```python
from build123d import *

# Parameters (mm, degrees)
SKETCH2_W         = 19.3548
SKETCH2_H         = 2.3876
SLOT_DEPTH        = 2.2352
SKETCH3_W         = 2.1844
SKETCH3_H         = 13.2842
SKETCH4_W         = 1.0922
SKETCH4_H         = 1.0922
CIRPATTERN1_COUNT = 2
CIRPATTERN1_ANGLE = 90


with BuildPart() as part:
    # BodySke → Base-Revolve (revolve)
    with BuildSketch(Plane.XY, mode=Mode.PRIVATE) as base_revolve_sk:
        Polygon((0, 0), (0, 9.6774), (0.066909223, 9.6774), (4.191, 4.7625), (38.1, 4.7625), (38.1, 0), align=None)
    revolve(base_revolve_sk.sketch.rotate(Axis((-6.35, 0, 0), (1, 0, 0)), 90), axis=Axis((-6.35, 0, 0), (1, 0, 0)))  # turned: the seam where the file's is

    # Sketch2 → Slot (cut)
    with BuildSketch(Plane.ZY):
        Rectangle(SKETCH2_W, SKETCH2_H)
    extrude(amount=-SLOT_DEPTH, mode=Mode.SUBTRACT)

    # Sketch3 → Cross section 0
    with BuildSketch(Plane.ZY):
        Rectangle(SKETCH3_W, SKETCH3_H)
    # Sketch4 → Cross section 1
    with BuildSketch(Plane.ZY.offset(-7.9756)):
        Rectangle(SKETCH4_W, SKETCH4_H)
    cross = loft(mode=Mode.SUBTRACT)

    # CirPattern1: Cross ×2 about axis
    cirpattern1_axis = Axis((0, 0, 0), (1, 0, 0))
    for i in range(1, CIRPATTERN1_COUNT):
        add(cross.rotate(cirpattern1_axis, i * CIRPATTERN1_ANGLE / (CIRPATTERN1_COUNT - 1)), mode=Mode.SUBTRACT)


solid = part.part
```
CAD build for the part. Positions are in the model's coordinates, mm. A direction names the side the tool comes from. Coordinates: 2 decimals unless noted, no trailing zeros. Order: outer loops, then holes, each group sorted by start corner. A loop starts at its lowest first (then second) coordinate and runs counter-clockwise, first axis right, second up. Notation, with made-up numbers: M 44.25,-32 L 92.25,-32 A27 ccw 92.25,6 Z; hole C 69.25,-4 d11. An arc over 180 degrees is marked long. Answer as CSV lines item,"result".
1) Mould opens along Y. For faces 3 (the flat face through (7.976, 0, 0)), 4 (the flat face through (1, -1.194, 4)), 5 (the cylindrical face through (21.38, 4.65, -1.03)), 6 (the flat face through (38.1, 0, 0)) say: released by +Y, released by -Y, zero draft, split by the parting line, or undercut.
Verdict:
face 3,"undercut"
face 4,"undercut"
face 5,"split by the parting line"
face 6,"zero draft"
2) Drill centre lines: L1, parallel to X at y = -0.25, z = 0.5; L2, parallel to X at y = -1, z = -2.25; L3, parallel to Y at x = 29, z = 0.25. Where is each one in solid material? Low to high. Write a range as from..to.
Verdict:
L1,"7.98..38.1"
L2,"2.24..38.1"
L3,"-4.76..4.76"
3) Flat gauge pins, fed straight in: P1, Ø6, axis at x = 19, z = 4.5, coming from the -Y side; P2, Ø3, axis at x = 13, y = -5.5, coming from the -Z side; P3, Ø1.8, axis at x = 1, z = 5, coming from the -Y side. Where does each tip first touch, or does it go through?
Verdict:
P1,"y = -4.52"
P2,"z = -2.58"
P3,"y = -8.35"
4) Cut at A-A (x = 31). List the corners of the cut face in (y, z) (1 decimal).
Verdict:
outline,"C 0,0 d9.5"
5) 3-axis set-ups, long thin cutter, end or side, ignore diameter. For faces 1 (the flat face through (0, 4, -2)), 2 (the flat face through (2.235, 0, -5.4)): which of +Z, -Z, +X, -X, +Y, -Y reach the whole face in a straight line?
Verdict:
face 1,"+Z, -Z, -X, +Y, -Y"
face 2,"+Z, -Z, -X"
